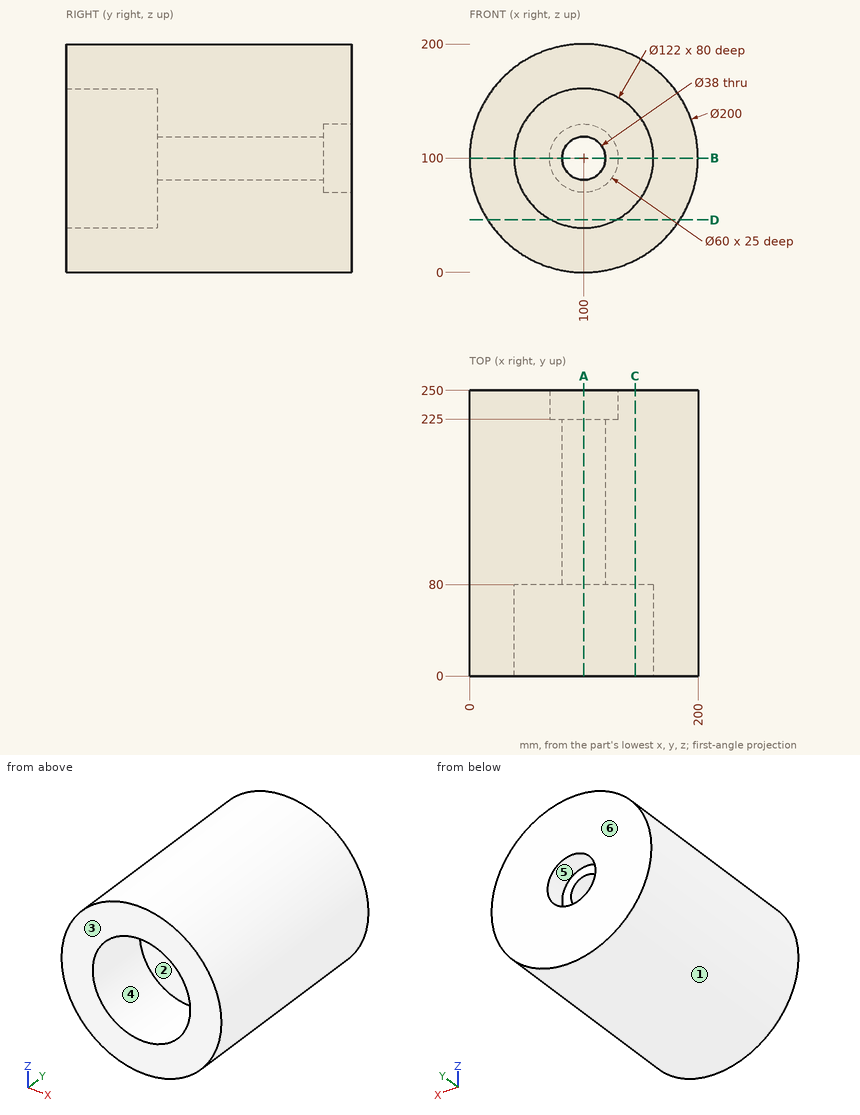
Print and shaded views of the part. All mm, measured from the part's lowest x, y and z. A direction names the side the tool comes from. Round coordinates to 2 decimals unless told otherwise and drop trailing zeros. Write each loop counter-clockwise with the first axis right and the second up, starting at its lowest first coordinate (ties: lowest second). Pieces come first, ordered by that corner, then holes. Notation, with made-up numbers: (80.25, -10.5) - (103.25, -10.5) arc R17 cw to (103.25, 19.5) - close; hole circle Ø7 at (-7, 0.25). An arc over 180 degrees is marked (long way). Use CSV: the item, a comma, the result in double quotes. Start each with the question number.
Item 1: Band-saw the part on A-A (x = 100). Write the cut outline in (y, z).
Item 2: Pin check, flat tips, straight feed: P1, Ø6, axis at x = 126.5, z = 101.5, coming from the -Y side; P2, Ø3, axis at x = 160, y = 218.5, coming from the +Z side; P3, Ø12, axis at x = 79, y = 73, coming from the -Z side. Stop position of each tip, or through.
Item 3: Band-saw the part on B-B (z = 100). Write the cut outline in (x, y), and give its area (3 significant figures).
Item 4: Band-saw the part on C-C (x = 145). Write the cut outline in (y, z).
Item 5: Drill centre lines: L1, parallel to Z at x = 100, y = 243; L2, parallel to Z at x = 100, y = 50.5; L3, parallel to Y at x = 136.5, z = 57. Where is each one in solid material? Low to high. Write a range as [from, to].
Item 6: Band-saw the part on D-D (z = 46). Write the cut outline in (x, y), and give its area (3 significant figures).
Item 7: Tool access for the marked faces 4, 5 and 6: list every direction of +Z, -Z, +X, -X, +Y, -Y with a clear straight run to the whole face (end or side of a thin tool).
Item 8: Two-plate mould, pull along X, no slides. Class the marked faces 1, 2 and 3: released by +X, released by -X, zero draft, split by the parting line, or undercut.
Checked values:
1,outline,"(0, 0) - (250, 0) - (250, 70) - (225, 70) - (225, 81) - (80, 81) - (80, 39) - (0, 39) - close; (0, 161) - (80, 161) - (80, 119) - (225, 119) - (225, 130) - (250, 130) - (250, 200) - (0, 200) - close"
2,P1,"stops at y = 80"
2,P2,"stops at z = 181.1"
2,P3,"stops at z = 1.13"
3,outline,"(0, 0) - (39, 0) - (39, 80) - (81, 80) - (81, 225) - (70, 225) - (70, 250) - (0, 250) - close; (119, 80) - (161, 80) - (161, 0) - (200, 0) - (200, 250) - (130, 250) - (130, 225) - (119, 225) - close"
3,area,"33,200 mm²"
4,outline,"(0, 10.7) - (250, 10.7) - (250, 189.3) - (0, 189.3) - (0, 141.18) - (80, 141.18) - (80, 58.82) - (0, 58.82) - close"
5,L1,"z = [0, 70], [130, 200]"
5,L2,"z = [0, 39], [161, 200]"
5,L3,"y = [80, 250]"
6,outline,"(15.83, 0) - (71.63, 0) - (71.63, 80) - (128.37, 80) - (128.37, 0) - (184.17, 0) - (184.17, 250) - (15.83, 250) - close"
6,area,"37,500 mm²"
7,face 4,"-Y"
7,face 5,"+Y"
7,face 6,"+Z, -Z, +X, -X, +Y"
8,face 1,"split by the parting line"
8,face 2,"undercut"
8,face 3,"zero draft"
